Part print with two shaded views. Sizes in mm from the minimum x, y, z corner. A direction names the side the tool comes from. Round coordinates to 2 decimals unless told otherwise and drop trailing zeros. Write each loop counter-clockwise with the first axis right and the second up, starting at its lowest first coordinate (ties: lowest second). Pieces come first, ordered by that corner, then holes. Notation, with made-up numbers: M 69.25,82 L 115.25,82 A20 cw 115.25,92 Z; hole C 3.25,81.25 d2. An arc over 180 degrees is marked long. Use one line per item in the form item = value. Start each with the question number.
Item 1: Cut at D-D, the plane y = 3.25. Give the cut face in (x, z).
Item 2: Flat gauge pins, fed straight in: pin 1 Ø4 at (y, z) = (7, 4) entering from -X; pin 2 Ø1.5 at (y, z) = (4.5, 21.5) entering from +X; pin 3 Ø2 at (x, y) = (13, 3.5) entering from +Z. Where does each tip first touch, or does it go through?
Item 3: Probe L1, parallel to Z at x = 23, y = 4; L2, parallel to X at y = 9.75, z = 14.5; L3, parallel to X at y = 6.5, z = 26.5. List the from-to ranges inside material, lowest first.
Item 4: Cut at B-B, the plane z = 16.35. Give the cut face in (x, y).
Item 5: Cut at C-C, the plane y = 6.35. Give the cut face in (x, z).
Item 6: Mould opens along Y. For the marked faces 4, 5 and 6 say: +Y half, -Y half, draft (parallel to the pull), parting line (faces both ways), or undercut.
Item 7: Which spindle directions (+Z, -Z, +X, -X, +Y, -Y) get a long thin tool onto all of the face, cutting with end or side? Do the marked faces 1, 2 and 3. Say none if no direction does.
Item 8: Cut at A-A, the plane x = 6.35. Give the cut face in (y, z).
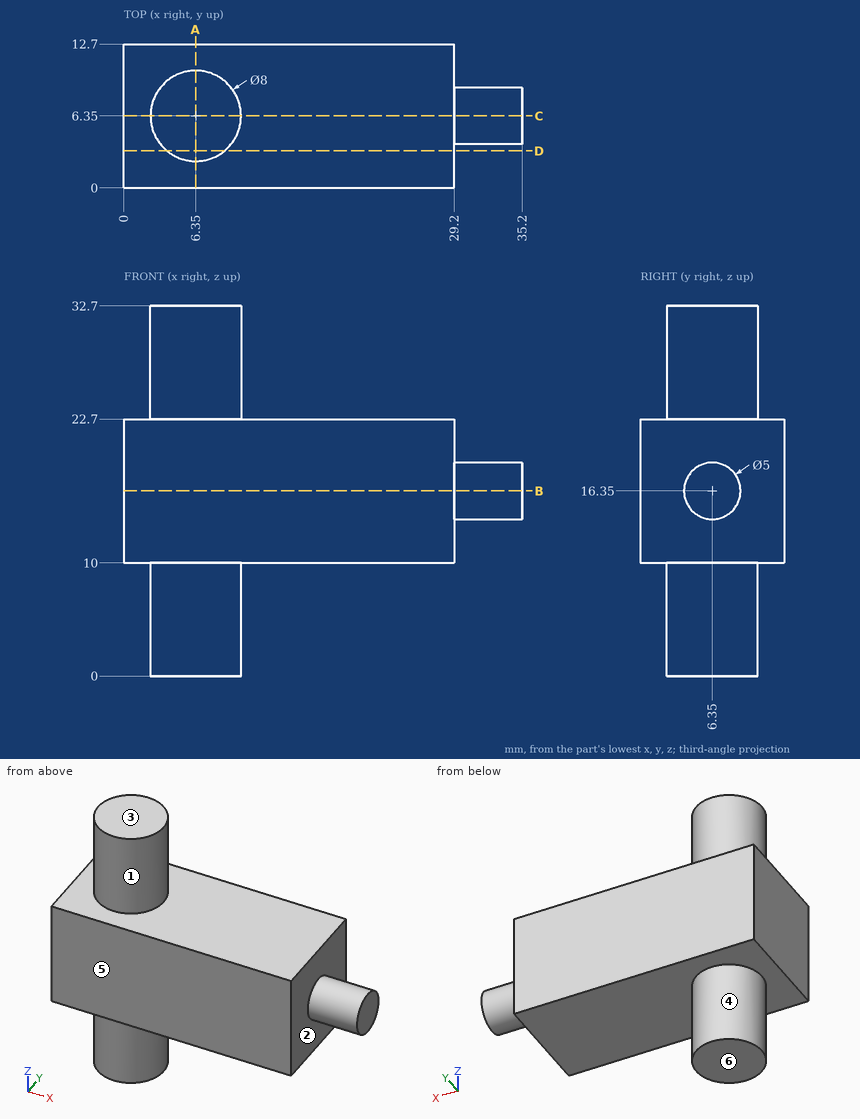
Model answer:
q1.outline = M 0,10 L 3.82,10 L 3.82,0 L 8.88,0 L 8.88,10 L 29.2,10 L 29.2,22.7 L 8.88,22.7 L 8.88,32.7 L 3.82,32.7 L 3.82,22.7 L 0,22.7 Z
q2.pin_1 = 2.35
q2.pin_2 = 29.2
q2.pin_3 = 22.7
q3.L1 = 10 to 22.7
q3.L2 = 0 to 29.2
q3.L3 = 2.35 to 10.35
q4.outline = M 0,0 L 29.2,0 L 29.2,3.85 L 35.2,3.85 L 35.2,8.85 L 29.2,8.85 L 29.2,12.7 L 0,12.7 Z
q5.outline = M 0,10 L 2.35,10 L 2.35,0 L 10.35,0 L 10.35,10 L 29.2,10 L 29.2,13.85 L 35.2,13.85 L 35.2,18.85 L 29.2,18.85 L 29.2,22.7 L 10.35,22.7 L 10.35,32.7 L 2.35,32.7 L 2.35,22.7 L 0,22.7 Z
q6.face_4 = parting line
q6.face_5 = -Y half
q6.face_6 = draft
q7.face_1 = +Z
q7.face_2 = +X
q7.face_3 = +Z, +X, -X, +Y, -Y
q8.outline = M 0,10 L 2.35,10 L 2.35,0 L 10.35,0 L 10.35,10 L 12.7,10 L 12.7,22.7 L 10.35,22.7 L 10.35,32.7 L 2.35,32.7 L 2.35,22.7 L 0,22.7 Z
